For this review, take the finished solid that the model builds, in its own axes (mm). A direction names the side the tool comes from. Coordinates: 2 decimals unless noted, no trailing zeros. Write each loop counter-clockwise with the first axis right and the second up, starting at its lowest first coordinate (ties: lowest second). Pieces come first, ordered by that corner, then holes. Notation, with made-up numbers: (25, -18) -> (34, -18) arc R27 cw to (34, 10) -> close; hole circle Ø6 at (-29.75, -15.5). An arc over 180 degrees is marked (long way). Put each result on its own line as item: value. Start each with the question number.
Item 1: Consider section C-C on y = 150. Give the boundary of the cut face in (x, z), and give its area (3 significant figures).
Item 2: For faces 1 (the flat face through (-36.83, 186, 1)), 2 (the cylindrical face through (-32.206, 13.137, 78.347)), list the 3-axis set-ups (+Z, -Z, +X, -X, +Y, -Y) from which the entire face can be reached by the end or side of a thin tool; tool diameter is ignored.
Item 3: To check wall thickness, follow L1, parallel to Y at x = -17.5, z = -8.5; L2, parallel to X at y = 260, z = 65; L3, parallel to Z at x = -40, y = 318. State the ranges of each line that lie inside material, in increasing order.
Item 4: Consider section A-A on z = -71.5. Give the boundary of the cut face in (x, y), and give its area (3 significant figures).
Item 5: Insertion check: P1, Ø4, axis at x = -30, z = -71, coming from the +Y side; P2, Ø1, axis at y = 228, z = 32, coming from the +X side; P3, Ø1, axis at x = -38, z = 11.5, coming from the -Y side; P4, Ø5, axis at x = -20.5, z = 81, coming from the +Y side. Each pin has a flat end and moves straight along its axis. Give the tip position at first contact, or say it passes through.
Item 6: Consider section B-B on x = -6.5. Give the boundary of the cut face in (y, z) (3 decimals).
```python
from build123d import *

# Parameters (mm, degrees)
EXTRUDE_THIN1_DEPTH     = 101.6
FILLET1_R               = 25.4
FILLET2_R               = 25.4
CUT_EXTRUDE1_DEPTH      = 15.494
CUT_EXTRUDE1_DEPTH_BACK = 67.818


with BuildPart() as part:
    # Sketch1 → Extrude-Thin1 (new, symmetric)
    with BuildSketch(Plane.XY):
        with BuildLine():
            Line((0, 0), (-19.05, 0))
            ThreePointArc((-19.05, 0), (-37.010512242, 7.439487758), (-44.45, 25.4))
            Line((-44.45, 25.4), (-44.45, 342.9))
            Line((-44.45, 342.9), (-36.83, 342.9))
            Line((-36.83, 342.9), (-36.83, 25.4))
            ThreePointArc((-36.83, 25.4), (-31.622358569, 12.827641431), (-19.05, 7.62))
            Line((-19.05, 7.62), (0, 7.62))
            Line((0, 7.62), (0, 0))
        make_face()
    extrude(amount=EXTRUDE_THIN1_DEPTH, both=True)

    # Fillet1
    fillet1_edges = [part.edges().sort_by_distance(p)[0] for p in [
        (-40.64, 342.9, 101.6),
    ]]
    fillet(fillet1_edges, radius=FILLET1_R)

    # Fillet2
    fillet2_edges = [part.edges().sort_by_distance(p)[0] for p in [
        (-40.64, 342.9, -101.6),
    ]]
    fillet(fillet2_edges, radius=FILLET2_R)

    # Sketch2 → Cut-Extrude1 (cut, two sides: drawn at the far end of the back side and taken through both)
    with BuildSketch(Plane(origin=(0, 0, 0), x_dir=(0, 0, -1), z_dir=(1, 0, 0)).offset(-CUT_EXTRUDE1_DEPTH_BACK)):
        with BuildLine():
            Line((-101.6, 0), (-76.2, 0))
            ThreePointArc((-76.2, 0), (-83.132124101, 22.895250599), (-101.6, 38.1))
            Line((-101.6, 38.1), (-101.6, 0))
        make_face()
        with BuildLine():
            Line((101.6, 0), (101.6, 38.1))
            ThreePointArc((101.6, 38.1), (83.132124101, 22.895250599), (76.2, 0))
            Line((76.2, 0), (101.6, 0))
        make_face()
    extrude(amount=CUT_EXTRUDE1_DEPTH + CUT_EXTRUDE1_DEPTH_BACK, mode=Mode.SUBTRACT)


solid = part.part
```
Return value:
1. outline: (-44.45, -101.6) -> (-36.83, -101.6) -> (-36.83, 101.6) -> (-44.45, 101.6) -> close
1. area: 1,550 mm^2
2. face 1: +Z, -Z, +X, +Y
2. face 2: +Z, +X, -X, -Y
3. L1: 0 to 7.62
3. L2: -44.45 to -36.83
3. L3: -101.6 to 101.6
4. outline: (-44.45, 25.4) arc R25.4 ccw to (-19.05, 0) -> (0, 0) -> (0, 7.62) -> (-19.05, 7.62) arc R17.78 cw to (-36.83, 25.4) -> (-36.83, 342.9) -> (-44.45, 342.9) -> close
4. area: 2,820 mm^2
5. P1: y = 13.22
5. P2: x = -36.83
5. P3: y = 7.94
5. P4: through
6. outline: (0, -76.2) arc R41.275 cw to (7.62, -76.909) -> (7.62, 76.909) arc R41.275 cw to (0, 76.2) -> close
